For this review, use the dimensioned drawing (mm, ordinates from the lowest corner) and the shaded views. A direction names the side the tool comes from. Give positions to 0.01 mm unless a question says otherwise; leave off trailing zeros. Write each loop counter-clockwise with the first axis right and the second up, starting at its lowest first coordinate (ties: lowest second). Pieces come first, ordered by that corner, then holes. Notation, with made-up numbers: (68.5, 5) -> (112.5, 5) arc R11 cw to (112.5, 10) -> close; hole circle Ø1 at (-0.75, -23). An arc over 180 degrees is marked (long way). Return JSON: item names as keys, results as strings.
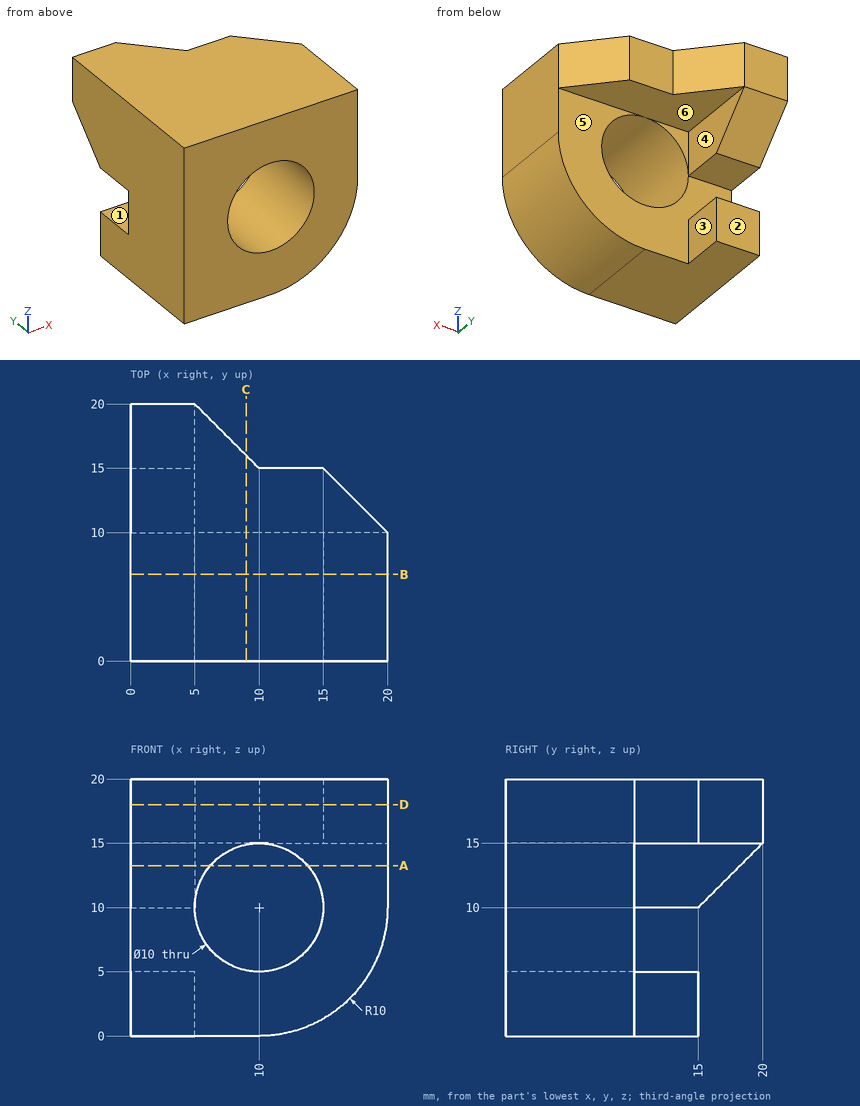
1. Add section A-A, the plane z = 13.25. State the section outline as (x, y) points.
Results found:
{"outline": "(0, 0) -> (6.2, 0) -> (6.2, 10) -> (5, 10) -> (5, 18.25) -> (0, 18.25) -> close; (13.8, 0) -> (20, 0) -> (20, 10) -> (13.8, 10) -> close"}
2. The part is to be moulded in two halves that separate along Z. For the marked faces 4, 5 and 6, say which applies: +Z half, -Z half, draft (parallel to the pull), parting line (faces both ways), or undercut.
Results found:
{"face 4": "draft", "face 5": "undercut", "face 6": "-Z half"}
3. Add section D-D, the plane z = 18. State the section outline as (x, y) points, plus the area to 3 significant figures.
Results found:
{"outline": "(0, 0) -> (20, 0) -> (20, 10) -> (15, 15) -> (10, 15) -> (5, 20) -> (0, 20) -> close", "area": "325 mm²"}
4. Add section C-C, the plane x = 9. State the section outline as (y, z) points, plus the area to 3 significant figures.
Results found:
{"outline": "(0, 0) -> (10, 0) -> (10, 5.1) -> (0, 5.1) -> close; (0, 14.9) -> (10, 14.9) -> (10, 15) -> (16, 15) -> (16, 20) -> (0, 20) -> close", "area": "132 mm²"}
5. For pin 1 (1.5 mm diameter, centred on x = 7.5, z = 13.5, fed in from +Y); pin 2 (5 mm diameter, centred on x = 14, y = 14.5, fed in from -Z); pin 3 (2.5 mm diameter, centred on y = 16.5, z = 12.5, fed in from +X), all flat-tipped, find the tip position at first contact; note any pin that passes through.
Results found:
{"pin 1": "stops at y = 10", "pin 2": "stops at z = 15", "pin 3": "stops at x = 5"}
6. Add section B-B, the plane y = 6.75. State the section outline as (x, z) points, plus the area to 3 significant figures.
Results found:
{"outline": "(0, 0) -> (10, 0) arc R10 ccw to (20, 10) -> (20, 20) -> (0, 20) -> close; hole circle Ø10 at (10, 10)", "area": "300 mm²"}
7. For the marked faces 1, 2 and 3, list the 3-axis set-ups (+Z, -Z, +X, -X, +Y, -Y) from which the entire face can be reached by the end or side of a thin tool; tool diameter is ignored.
Results found:
{"face 1": "+X, -X, +Y", "face 2": "-Z, +X, -X, +Y", "face 3": "-Z, +X, +Y"}
8. To check wall thickness, follow probe 1 along X at (y, z) = (3.5, 10); probe 2 along Y at (x, z) = (18.25, 12). State the ranges of each line that lie inside material, in increasing order.
Results found:
{"probe 1": "x = 0 to 5, 15 to 20", "probe 2": "y = 0 to 10"}
